Autodesk Inventor part; units mm, degrees
ref_plane "YZ Plane" through (0, 0, 0) normal (1, 0, 0) x (0, 1, 0)
ref_plane "XZ Plane" through (0, 0, 0) normal (0, 1, 0) x (-1, 0, 0)
ref_plane "XY Plane" through (0, 0, 0) normal (0, 0, 1) x (1, 0, 0)
sketch "Sketch1" plane through (0, 0, 0) normal (0, 0, 1) x (1, 0, 0)
  circle A0 centre (14.3651, 1.9735) radius 1.5
  circle A1 centre (14.3651, 1.9735) radius 5
  circle A2 centre (14.3651, 1.9735) radius 1.5
  point P0 (0, 0)
  dimension "d0" = 10
  dimension "d1" = 3
extrude "Extrusion1" add sketch "Sketch1" along normal blind 5
sketch "Sketch2" plane through (14.3651, 1.9735, 5) normal (0, 0, 1) x (1, 0, 0)
  circle A0 centre (0, 0) radius 5
  circle A1 centre (0, 0) radius 1.5
  circle A2 centre (0, 0) radius 2
  circle A3 centre (0, 0) radius 4
  point P0 (-14.3651, -1.9735)
  dimension "d4" = 4
  dimension "d5" = 8
extrude "Extrusion2" cut sketch "Sketch2" against normal blind 0.1 contours A3
sketch "Sketch3" plane through (14.3651, 1.9735, 0) normal (0, 0, -1) x (-1, 0, 0)
  circle A0 centre (0, 0) radius 4
  circle A1 centre (0, 0) radius 2
  point P0 (14.3651, -1.9735)
extrude "Extrusion3" cut sketch "Sketch3" against normal blind 0.1
properties part number "bearing_3_10_5"
Verification items for the finished model (mm, model axes). A direction names the side the tool comes from. Round coordinates to 2 decimals unless told otherwise and drop trailing zeros. Loops run counter-clockwise (first coordinate to the right, second up) from the corner with the lowest first, then second, coordinate; pieces in that order, holes last. Notation, with made-up numbers: (62, -2.75) - (92, -2.75) arc R28 ccw to (92, 22.25) - close; hole circle Ø4 at (80.25, 3). An arc over 180 degrees is marked (long way). Answer in a Markdown table with one row per item. Add a question column.
Q1. Section check A-A on x = 14. Enter the section's corners in (y, z), plus the area to 3 significant figures.
Q2. Section check D-D on z = 2.55. Enter the section's corners in (x, y).
Q3. Material ranges on line 1 (Z direction, x = 11, y = 1.75); line 2 (Y direction, x = 13.25, z = 1.1); line 3 (Y direction, x = 13.5, z = 1.2), recorded low to high.
Q4. Release check for a two-part mould opening along X. For faces 1 (the face through (16, 6, 0)), 2 (the face through (13, 0, 0.1)), 3 (the face through (13.714, -2.984, 2.465)) record: pulls with the +X half, pulls with the -X half, needs draft (parallel to the pull), parting line crosses it, or undercut.
Q5. Section check B-B on y = 1.5. Enter the section's corners in (x, z), plus the area to 3 significant figures.
Q6. Section check C-C on x = 17. Enter the section's corners in (y, z).
Q7. Gauge pin test, flat ends, axial feed: pin 1 (2 mm diameter, centred on x = 18, z = 0.5, fed in from +Y); pin 2 (1.8 mm diameter, centred on x = 14.37, y = 1.97, fed in from -Z); pin 3 (1 mm diameter, centred on x = 11, z = 0.5, fed in from +Y); pin 4 (1.5 mm diameter, centred on x = 17.5, z = 3, fed in from +Y). Record the tip position at first contact, or that the pin passes through.
Q8. Tool access check on faces 4 (the face through (13, 3, 5)), 5 (the face through (13, 4, 4.9)). Record the directions out of +Z, -Z, +X, -X, +Y, -Y that give a thin tool (end or side, any length) a straight path to the whole face; none if there is none.
Found:
| question | item | result |
|---|---|---|
| 1 | outline | (-3.01, 0) - (-2.01, 0) - (-2.01, 0.1) - (0.01, 0.1) - (0.01, 0) - (0.52, 0) - (0.52, 5) - (0.01, 5) - (0.01, 4.9) - (-2.01, 4.9) - (-2.01, 5) - (-3.01, 5) - close; (3.43, 0) - (3.94, 0) - (3.94, 0.1) - (5.96, 0.1) - (5.96, 0) - (6.96, 0) - (6.96, 5) - (5.96, 5) - (5.96, 4.9) - (3.94, 4.9) - (3.94, 5) - (3.43, 5) - close |
| 1 | area | 34.5 mm² |
| 2 | outline | circle Ø10 at (14.37, 1.97); hole circle Ø3 at (14.37, 1.97) |
| 3 | line 1 | z = 0.1 to 4.9 |
| 3 | line 2 | y = -2.9 to 0.97, 2.98 to 6.85 |
| 3 | line 3 | y = -2.95 to 0.75, 3.2 to 6.9 |
| 4 | face 1 | needs draft |
| 4 | face 2 | undercut |
| 4 | face 3 | parting line crosses it |
| 5 | outline | (9.39, 0) - (10.39, 0) - (10.39, 0.1) - (12.42, 0.1) - (12.42, 0) - (12.94, 0) - (12.94, 5) - (12.42, 5) - (12.42, 4.9) - (10.39, 4.9) - (10.39, 5) - (9.39, 5) - close; (15.79, 0) - (16.31, 0) - (16.31, 0.1) - (18.34, 0.1) - (18.34, 0) - (19.34, 0) - (19.34, 5) - (18.34, 5) - (18.34, 4.9) - (16.31, 4.9) - (16.31, 5) - (15.79, 5) - close |
| 5 | area | 34.7 mm² |
| 6 | outline | (-2.28, 0) - (-1.04, 0) - (-1.04, 0.1) - (4.98, 0.1) - (4.98, 0) - (6.22, 0) - (6.22, 5) - (4.98, 5) - (4.98, 4.9) - (-1.04, 4.9) - (-1.04, 5) - (-2.28, 5) - close |
| 7 | pin 1 | stops at y = 6.22 |
| 7 | pin 2 | passes through |
| 7 | pin 3 | stops at y = 6.07 |
| 7 | pin 4 | stops at y = 6.37 |
| 8 | face 4 | +Z, +X, -X, +Y, -Y |
| 8 | face 5 | +Z |
